Design review of the part built by this model. Coordinates are the model's own, in mm. Face numbers are marked on the shaded views. A direction names the side the tool comes from. Round coordinates to 2 decimals unless told otherwise and drop trailing zeros. Order: outer loops, then holes, each group sorted by start corner. A loop starts at its lowest first (then second) coordinate and runs counter-clockwise, first axis right, second up.
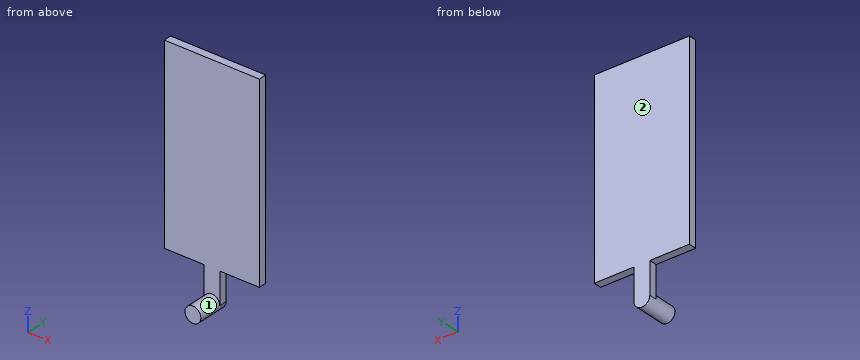
from build123d import *

# Parameters (mm, degrees)
F1_DEPTH = 6.35
F2_DEPTH = 25.4


with BuildPart() as f1:
    # F0 (on Front) → F1 (new body)
    with BuildSketch(Plane.XZ):
        Polygon((6.35, -76.2), (38.1, -76.2), (38.1, 76.2), (-38.1, 76.2), (-38.1, -76.2), (-6.35, -76.2), align=None)
        with BuildLine():
            Line((6.35, -101.6), (6.35, -76.2))
            Line((6.35, -76.2), (-6.35, -76.2))
            Line((-6.35, -76.2), (-6.35, -101.6))
            ThreePointArc((-6.35, -101.6), (0, -95.25), (6.35, -101.6))
        make_face()
    extrude(amount=F1_DEPTH)

    # F0 (on Front) → F2 (join)
    with BuildSketch(Plane.XZ):
        with BuildLine():
            ThreePointArc((-6.35, -101.6), (0, -107.95), (6.35, -101.6))
            ThreePointArc((6.35, -101.6), (0, -95.25), (-6.35, -101.6))
        make_face()
    extrude(amount=F2_DEPTH)


solid = f1.part
1) Take a section at D-D on x = 14.5. Give the boundary of the cut face in (y, z).
Results:
outline: (-6.35, -76.2) - (0, -76.2) - (0, 76.2) - (-6.35, 76.2) - close
2) Clearance check with flat-ended pins moving along their axes: P1, Ø3, axis at x = 18.5, y = -2, coming from the -Z side; P2, Ø3, axis at y = -2, z = -93, coming from the -X side; P3, Ø1.9, axis at y = -2, z = -90.5, coming from the +X side. State where each tip first meets the part, or that it passes through.
Results:
P1: stops at z = -76.2
P2: stops at x = -6.35
P3: stops at x = 6.35
3) To check wall thickness, follow line 1 along Y through (x, z) = (3, -77.5); line 2 along Z through (x, y) = (-25, -2.5); line 3 along X through (y, z) = (-15.25, -98). State the ranges of each line that lie inside material, in increasing order.
Results:
line 1: y = -6.35 to 0
line 2: z = -76.2 to 76.2
line 3: x = -5.23 to 5.23
4) Take a section at B-B on y = -17. Give the boundary of the cut face in (x, z).
Results:
outline: circle Ø12.7 at (0, -101.6)
5) Take a section at A-A on x = 0. Give the boundary of the cut face in (y, z), plus the area to 3 significant figures.
Results:
outline: (-25.4, -107.95) - (0, -107.95) - (0, 76.2) - (-6.35, 76.2) - (-6.35, -95.25) - (-25.4, -95.25) - close
area: 1,410 mm2
6) For the marked faces 1 and 2, list the 3-axis set-ups (+Z, -Z, +X, -X, +Y, -Y) from which the entire face can be reached by the end or side of a thin tool; tool diameter is ignored.
Results:
face 1: -Y
face 2: +Z, -Z, +X, -X, +Y
7) Take a section at C-C on z = -45.5. Give the boundary of the cut face in (x, y).
Results:
outline: (-38.1, -6.35) - (38.1, -6.35) - (38.1, 0) - (-38.1, 0) - close
